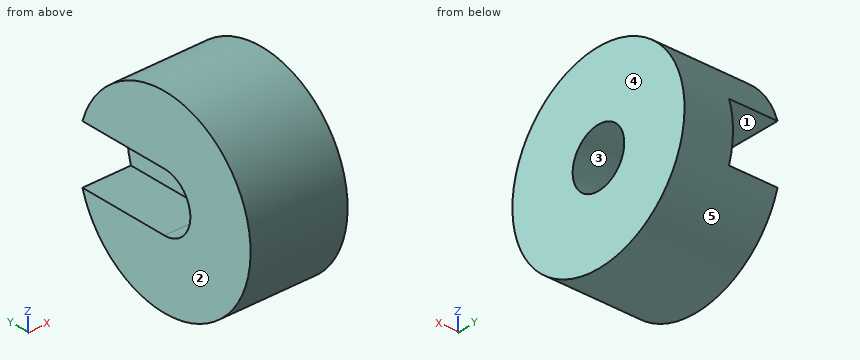
```python
from build123d import *

# Parameters (mm, degrees)
SKETCH_1_R          = 10
SKETCH_1_R_2        = 3
EXTRUDE_1_DEPTH     = 10
CUT_EXTRUDE_1_DEPTH = 5


with BuildPart() as part:
    # ｽｹｯﾁ1 → ﾎﾞｽ - 押し出し1 (new body)
    with BuildSketch(Plane(origin=(0, 0, 0), x_dir=(0, 0, -1), z_dir=(1, 0, 0))):
        Circle(SKETCH_1_R)
        Circle(SKETCH_1_R_2, mode=Mode.SUBTRACT)
    extrude(amount=EXTRUDE_1_DEPTH)

    # ｽｹｯﾁ2 → ｶｯﾄ - 押し出し1 (cut)
    with BuildSketch(Plane.ZY):
        with BuildLine():
            Line((3, 10), (3, 0))
            ThreePointArc((3, 0), (0, -3), (-3, 0))
            Line((-3, 0), (-3, 10))
            ThreePointArc((-3, 10), (0, 13), (3, 10))
        make_face()
    extrude(amount=-CUT_EXTRUDE_1_DEPTH, mode=Mode.SUBTRACT)


solid = part.part
```
Could you check a few things on this model? Use its own coordinates, in mm. Face numbers are marked on the shaded views. A direction names the side the tool comes from. Give positions to 0.01 mm unless a question says otherwise; leave off trailing zeros. Loops run counter-clockwise (first coordinate to the right, second up) from the corner with the lowest first, then second, coordinate; pieces in that order, holes last. Notation, with made-up numbers: (82.25, 31) - (141.25, 31) arc R19 ccw to (141.25, 44) - close; hole circle Ø6 at (52.25, 42.5). An arc over 180 degrees is marked (long way). Answer in a Markdown table with one row per item. Add a question column.
Q1. If we section it at B-B (y = 4): List the corners of the cut face in (x, z) for me.
Q2. For pin 1 (6.5 mm diameter, centred on y = 5, z = -1, fed in from -X); pin 2 (4 mm diameter, centred on x = 1, z = -7, fed in from +Y); pin 3 (5.5 mm diameter, centred on x = 2.5, y = 4, fed in from +Z); pin 4 (4 mm diameter, centred on x = 3.5, z = -7, fed in from -Y), each with a flat end and sliding along its axis, tell me the tip position at first contact or that it passes through.
Q3. If we section it at A-A (z = 0): List the corners of the cut face in (x, y) for me, plus the area to 3 significant figures.
Q4. Which directions (+Z, -Z, +X, -X, +Y, -Y) give clear straight access to the entire face, cutting with the end or side of a thin tool? Please do the marked faces 1 and 2.
Q5. If we section it at D-D (z = 3.75): List the corners of the cut face in (x, y) for me, plus the area to 3 significant figures.
Q6. Please list where these lines run through material, in increasing order: L1, parallel to Z at x = 6.75, y = 0; L2, parallel to Z at x = 3.5, y = 7.75; L3, parallel to Y at x = 2.75, z = 0. Write a range as from..to.
Q7. If we section it at C-C (x = 2.5): List the corners of the cut face in (y, z) for me, plus the area to 3 significant figures.
Q8. We'd pull the mould along Z, two halves only. Please class the marked faces 3, 4 and 5: +Z half, -Z half, draft (parallel to the pull), parting line (faces both ways), or undercut.
The answers:
| question | item | result |
|---|---|---|
| 1 | outline | (0, -9.17) - (10, -9.17) - (10, 9.17) - (0, 9.17) - (0, 3) - (5, 3) - (5, -3) - (0, -3) - close |
| 2 | pin 1 | stops at x = 0 |
| 2 | pin 2 | stops at y = 8.66 |
| 2 | pin 3 | stops at z = 9.92 |
| 2 | pin 4 | stops at y = -8.66 |
| 3 | outline | (0, -10) - (10, -10) - (10, -3) - (0, -3) - close; (5, 3) - (10, 3) - (10, 10) - (5, 10) - close |
| 3 | area | 105 mm^2 |
| 4 | face 1 | -X, +Y |
| 4 | face 2 | +Z, -Z, -X, +Y, -Y |
| 5 | outline | (0, -9.27) - (10, -9.27) - (10, 9.27) - (0, 9.27) - close |
| 5 | area | 185 mm^2 |
| 6 | L1 | z = -10..-3, 3..10 |
| 6 | L2 | z = -6.32..-3, 3..6.32 |
| 6 | L3 | y = -10..-3 |
| 7 | outline | (0, -3) arc R3 cw to (0, 3) - (9.54, 3) arc R10 ccw (long way) to (9.54, -3) - close |
| 7 | area | 241 mm^2 |
| 8 | face 3 | undercut |
| 8 | face 4 | draft |
| 8 | face 5 | parting line |
